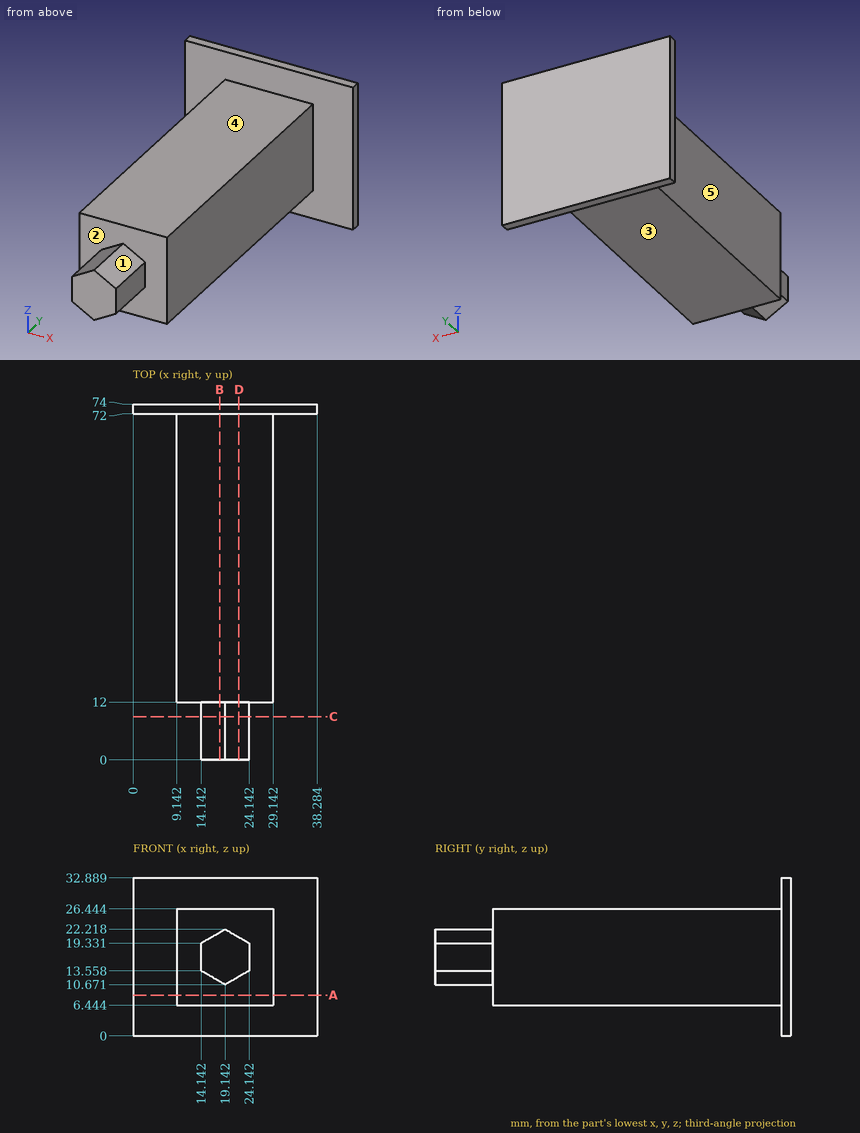
Here's the drawing with two shaded views (mm, measured from the low corner). I have some questions. A direction names the side the tool comes from. Coordinates: 2 decimals unless noted, no trailing zeros. Loops run counter-clockwise (first coordinate to the right, second up) from the corner with the lowest first, then second, coordinate; pieces in that order, holes last. Notation, with made-up numbers: (-15.5, 69.25) -> (11.5, 69.25) arc R30 ccw to (11.5, 96.25) -> close; hole circle Ø8 at (57.5, 7.25). An arc over 180 degrees is marked (long way). Answer as a JSON object with one key per item and string values.
1) Imagine slicing it at B-B (x = 18). Please give me the cut outline in (y, z) (1 decimal), then the cut area to 3 significant figures.
Results:
{"outline": "(0, 11.3) -> (12, 11.3) -> (12, 6.4) -> (72, 6.4) -> (72, 0) -> (74, 0) -> (74, 32.9) -> (72, 32.9) -> (72, 26.4) -> (12, 26.4) -> (12, 21.6) -> (0, 21.6) -> close", "area": "1,390 mm^2"}
2) Imagine slicing it at A-A (z = 8.5). Please give me the cut outline in (x, y) (1 decimal).
Results:
{"outline": "(0, 72) -> (9.1, 72) -> (9.1, 12) -> (29.1, 12) -> (29.1, 72) -> (38.3, 72) -> (38.3, 74) -> (0, 74) -> close"}
3) For P1, Ø6.5, axis at y = 8, z = 16.5, coming from the +X side; P2, Ø16, axis at y = 33, z = 14, coming from the +X side; P3, Ø12, axis at x = 4, y = 25.5, coming from the -Z side, each with a flat end and sliding along its axis, tell me the tip position at first contact or that it passes through.
Results:
{"P1": "stops at x = 24.14", "P2": "stops at x = 29.14", "P3": "stops at z = 6.44"}
4) Imagine slicing it at C-C (y = 9). Please give me the cut outline in (x, z), then the cut area to 3 significant figures.
Results:
{"outline": "(14.14, 13.56) -> (19.14, 10.67) -> (24.14, 13.56) -> (24.14, 19.33) -> (19.14, 22.22) -> (14.14, 19.33) -> close", "area": "86.6 mm^2"}
5) If I drill on line 1 (Y direction, x = 7, z = 31.5); line 2 (Z direction, x = 10, y = 46) (1 decimal); line 3 (Y direction, x = 25, z = 14.5), over which ranges is the centre line in solid material (lowest first)?
Results:
{"line 1": "y = 72 to 74", "line 2": "z = 6.4 to 26.4", "line 3": "y = 12 to 74"}
6) Imagine slicing it at D-D (x = 22). Please give me the cut outline in (y, z) (1 decimal).
Results:
{"outline": "(0, 12.3) -> (12, 12.3) -> (12, 6.4) -> (72, 6.4) -> (72, 0) -> (74, 0) -> (74, 32.9) -> (72, 32.9) -> (72, 26.4) -> (12, 26.4) -> (12, 20.6) -> (0, 20.6) -> close"}
7) For the marked faces 1, 2, 3, 4 and 5, which set-ups out of +Z, -Z, +X, -X, +Y, -Y let a thin tool reach every point of the face, with its end or its side?
Results:
{"face 1": "+Z, +X, -Y", "face 2": "-Y", "face 3": "-Z, +X, -X, -Y", "face 4": "+Z, +X, -X, -Y", "face 5": "+Z, -Z, -X, -Y"}
